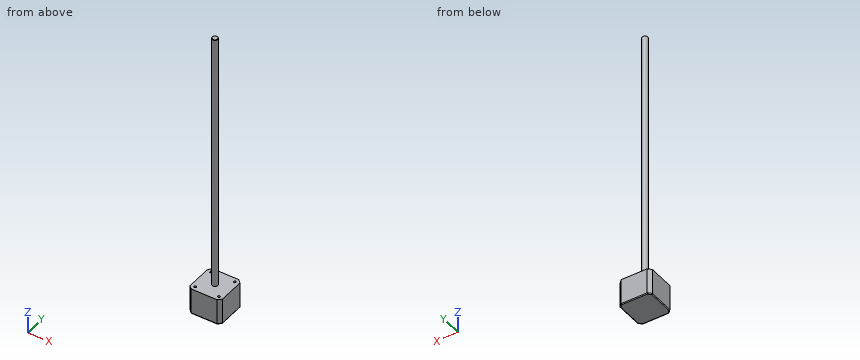
```python
from build123d import *

# Parameters (mm, degrees)
SKETCH_W        = 41
SKETCH_H        = 41
PAD_DEPTH       = 33
CHAMFER_SIZE    = 4
FILLET_R        = 1
SKETCH001_R     = 1.5
POCKET_DEPTH    = 5
SKETCH002_R     = 3.75
PAD001_DEPTH    = 330
CHAMFER001_SIZE = 0.5


with BuildPart() as part:
    # Sketch → Pad (new body)
    with BuildSketch(Plane.XY):
        with Locations((20.5, 20.5)):
            Rectangle(SKETCH_W, SKETCH_H)
    extrude(amount=PAD_DEPTH)

    # Chamfer
    chamfer_edges = [part.edges().sort_by_distance(p)[0] for p in [
        (41, 0, 16.5),
        (0, 0, 16.5),
        (0, 41, 16.5),
        (41, 41, 16.5),
    ]]
    chamfer(chamfer_edges, length=CHAMFER_SIZE)

    # Fillet
    fillet_edges = [part.edges().sort_by_distance(p)[0] for p in [
        (20.5, 0, 0),
        (39, 2, 0),
        (41, 20.5, 0),
        (39, 39, 0),
        (20.5, 41, 0),
        (2, 39, 0),
        (0, 20.5, 0),
        (2, 2, 0),
    ]]
    fillet(fillet_edges, radius=FILLET_R)

    # Sketch001 (on Face4 of Fillet) → Pocket (cut)
    with BuildSketch(Plane.XY.offset(33)):
        with Locations((35.5, 35.5)):
            Circle(SKETCH001_R)
        with Locations((5.5, 35.5)):
            Circle(SKETCH001_R)
        with Locations((5.5, 5.5)):
            Circle(SKETCH001_R)
        with Locations((35.5, 5.5)):
            Circle(SKETCH001_R)
    extrude(amount=-POCKET_DEPTH, mode=Mode.SUBTRACT)

    # Sketch002 (on Face4 of Pocket) → Pad001 (join)
    with BuildSketch(Plane.XY.offset(33)):
        with Locations((20.5, 20.5)):
            Circle(SKETCH002_R)
    extrude(amount=PAD001_DEPTH)

    # Chamfer001
    chamfer001_edges = [part.edges().sort_by_distance(p)[0] for p in [
        (16.75, 20.5, 363),
    ]]
    chamfer(chamfer001_edges, length=CHAMFER001_SIZE)


solid = part.part
```
Verification items for the finished model (mm, model axes). Round coordinates to 2 decimals unless told otherwise and drop trailing zeros. Write each loop counter-clockwise with the first axis right and the second up, starting at its lowest first coordinate (ties: lowest second). Pieces come first, ordered by that corner, then holes.
1. Scan lines: L1, parallel to Y at x = 35.5, z = 31.4; L2, parallel to Z at x = 2.5, y = 23; L3, parallel to Y at x = 22.5, z = 106.5. Record each from-to range of solid material in increasing order.
2. Section check C-C on z = 256. Enter the section's corners in (x, y).
3. Section check A-A on x = 20.5. Enter the section's corners in (y, z), plus the area to 3 significant figures.
4. Gauge pin test, flat ends, axial feed: P1, Ø4, axis at x = 31.5, y = 23.5, coming from the +Z side; P2, Ø0.9, axis at x = 35, y = 35, coming from the +Z side; P3, Ø1.5, axis at y = 21.5, z = 264.5, coming from the -X side; P4, Ø6, axis at y = 27.5, z = 213.5, coming from the +X side. Record the tip position at first contact, or that the pin passes through.
Answer:
1. L1: y = 0 to 4, 7 to 34, 37 to 41
1. L2: z = 0 to 33
1. L3: y = 17.33 to 23.67
2. outline: circle Ø7.5 at (20.5, 20.5)
3. outline: (0, 1) arc R1 ccw to (1, 0) - (40, 0) arc R1 ccw to (41, 1) - (41, 33) - (24.25, 33) - (24.25, 362.5) - (23.75, 363) - (17.25, 363) - (16.75, 362.5) - (16.75, 33) - (0, 33) - close
3. area: 3,830 mm2
4. P1: stops at z = 33
4. P2: stops at z = 28
4. P3: stops at x = 16.76
4. P4: passes through
